Read the model definition and answer for the solid it produces. Units are mm, in the model's axes. Face numbers are marked on the shaded views. A direction names the side the tool comes from. Coordinates: 2 decimals unless noted, no trailing zeros. Loops run counter-clockwise (first coordinate to the right, second up) from the corner with the lowest first, then second, coordinate; pieces in that order, holes last. Notation, with made-up numbers: M 46.5,32 L 56.5,32 A8 ccw 56.5,41 Z; hole C 73,28 d11. An arc over 180 degrees is marked long. Put each result on its own line as item: value.
from build123d import *

# Parameters (mm, degrees)
F0_W     = 215
F0_H     = 65
F1_DEPTH = 2.5
F2_DEPTH = 19.05
F3_R     = 5.08


with BuildPart() as f1:
    # F0 (on Top) → F1 (new body)
    with BuildSketch(Plane.XY):
        with Locations((21.428473, -29.951386)):
            Rectangle(F0_W, F0_H)
    extrude(amount=F1_DEPTH)

    # F0 (on Top) → F2 (join, symmetric)
    with BuildSketch(Plane.XY):
        with BuildLine():
            Line((128.928473, -62.451386), (-86.071527, -62.451386))
            Line((-86.071527, -62.451386), (-88.571527, -62.451386))
            Line((-88.571527, -62.451386), (-88.571527, -86.101386))
            ThreePointArc((-88.571527, -86.101386), (-86.711655, -90.591514), (-82.221527, -92.451386))
            Line((-82.221527, -92.451386), (125.078473, -92.451386))
            ThreePointArc((125.078473, -92.451386), (129.568601, -90.591514), (131.428473, -86.101386))
            Line((131.428473, -86.101386), (131.428473, -62.451386))
            Line((131.428473, -62.451386), (128.928473, -62.451386))
        make_face()
    extrude(amount=F2_DEPTH, both=True)

    # F3
    f3_edges = [f1.edges().sort_by_distance(p)[0] for p in [
        (21.428473, -92.451386, 19.05),
        (21.428473, -92.451386, -19.05),
        (21.428473, -62.451386, 19.05),
        (21.428473, -62.451386, -19.05),
    ]]
    fillet(f3_edges, radius=F3_R)


solid = f1.part
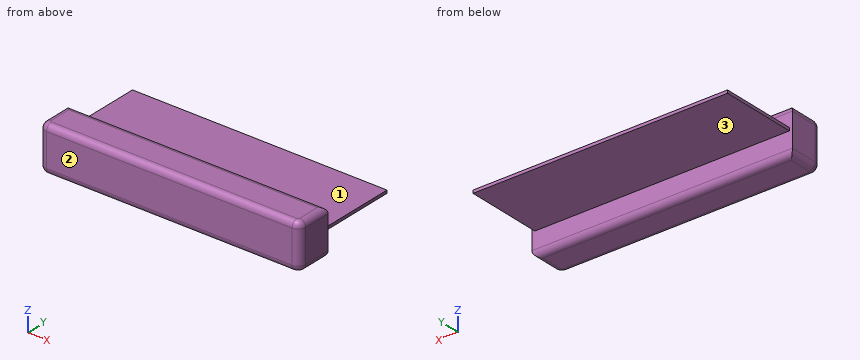
1) Straight lines are drawn through the part: line 1 (Z direction, x = 91.5, y = -87.5); line 2 (Y direction, x = 119.5, z = 13); line 3 (Y direction, x = -44, z = -14.5). For each, find the intervals that lie inside material, in ascending order. Write a range as [from, to].
Answer list:
line 1: z = [-19.05, 19.05]
line 2: y = [-92.45, -62.45]
line 3: y = [-92.42, -62.48]
2) Find section B-B, the plane z = 10. Write down the section's boundary in (x, y).
Answer list:
outline: M -88.57,-86.1 A6.35 ccw -82.22,-92.45 L 125.08,-92.45 A6.35 ccw 131.43,-86.1 L 131.43,-62.45 L -88.57,-62.45 Z
3) Given pin 1 Ø4 at (x, y) = (-25, -47.5) entering from +Z; pin 2 Ø3 at (x, y) = (-60.5, -14.5) entering from -Z; pin 3 Ø8 at (y, z) = (-50, -2.5) entering from -X, each flat-ended and moving along its own axis, determine where each tip first touches the part or whether it passes through.
Answer list:
pin 1: stops at z = 2.5
pin 2: stops at z = 0
pin 3: stops at x = -86.07
4) Find section C-C, the plane y = -41. Write down the section's boundary in (x, z), plus the area to 4 significant figures.
Answer list:
outline: M -86.07,0 L 128.93,0 L 128.93,2.5 L -86.07,2.5 Z
area: 537.5 mm^2
5) Which of the six approach directions +Z, -Z, +X, -X, +Y, -Y give full straight-line access (tool end or side, diameter ignored) to the marked faces 1, 2 and 3?
Answer list:
face 1: +Z, +X, -X, +Y
face 2: +Z, -Z, +X, -X, -Y
face 3: -Z, +X, -X, +Y
6) Find section A-A, the plane x = 52. Write down the section's boundary in (y, z).
Answer list:
outline: M -92.45,-13.97 A5.08 ccw -87.37,-19.05 L -67.53,-19.05 A5.08 ccw -62.45,-13.97 L -62.45,0 L 2.55,0 L 2.55,2.5 L -62.45,2.5 L -62.45,13.97 A5.08 ccw -67.53,19.05 L -87.37,19.05 A5.08 ccw -92.45,13.97 Z
